from build123d import *

# Parameters (mm, degrees)
EXTRUDE1_DEPTH      = 3.175
SKETCH3_R           = 2.0955
EXTRUDE2_DEPTH      = 4.175
CIRPATTERN1_COUNT   = 10
CIRPATTERN1_ANGLE   = 35
EXTRUDE3_DEPTH      = 1
EXTRUDE3_DEPTH_BACK = 4.175
SKETCH5_W           = 1.778
SKETCH5_H           = 1.961783436
EXTRUDE4_DEPTH      = 4.175


with BuildPart() as part:
    # Sketch1 → Extrude1 (new body)
    with BuildSketch(Plane.XY):
        with BuildLine():
            Line((0, 0), (228.6, 0))
            Line((228.6, 0), (228.6, 90.4875))
            ThreePointArc((228.6, 90.4875), (105.671212021, 67.042793316), (0, 0))
        make_face()
        with BuildLine():
            Line((40.029392194, 9.525), (209.55, 9.525))
            ThreePointArc((209.55, 9.525), (216.285192091, 12.314807909), (219.075, 19.05))
            Line((219.075, 19.05), (219.075, 74.358899247))
            ThreePointArc((219.075, 74.358899247), (218.099794794, 76.648337576), (215.773250164, 77.531368235))
            ThreePointArc((215.773250164, 77.531368235), (122.297861029, 59.693048715), (38.147400573, 15.25709455))
            ThreePointArc((38.147400573, 15.25709455), (37.012821277, 11.709583471), (40.029392194, 9.525))
        make_face(mode=Mode.SUBTRACT)
    extrude(amount=EXTRUDE1_DEPTH)

    # Sketch3 → Extrude2 (cut, through all)
    with BuildSketch(Plane.XY.offset(3.175)):
        with Locations((15.875, 7.775506467)):
            Circle(SKETCH3_R)
    extrude2 = extrude(amount=-EXTRUDE2_DEPTH, mode=Mode.SUBTRACT)

    # CirPattern1: Extrude2 ×10 about axis
    cirpattern1_axis = Axis((228.6, -243.514144737, 0), (0, 0, -1))
    for i in range(1, CIRPATTERN1_COUNT):
        add(extrude2.rotate(cirpattern1_axis, i * CIRPATTERN1_ANGLE / (CIRPATTERN1_COUNT - 1)), mode=Mode.SUBTRACT)

    # Sketch4 → Extrude3 (cut, two sides)
    with BuildSketch(Plane.XY.offset(3.175)) as extrude3_sk:
        with BuildLine():
            Line((726.667212815, 85.4075), (228.6, 85.4075))
            ThreePointArc((228.6, 85.4075), (107.540898152, 62.319375722), (3.476893058, -3.703729831))
            Line((3.476893058, -3.703729831), (-359.654286867, -344.594760291))
            Line((-359.654286867, -344.594760291), (6.971445482, -1270.807136749))
            Line((6.971445482, -1270.807136749), (1093.292945163, -840.804876459))
            Line((1093.292945163, -840.804876459), (726.667212815, 85.4075))
        make_face()
    extrude(amount=EXTRUDE3_DEPTH, mode=Mode.SUBTRACT)
    extrude(extrude3_sk.sketch, amount=-EXTRUDE3_DEPTH_BACK, mode=Mode.SUBTRACT)

    # Sketch5 → Extrude4 (cut, through all)
    with BuildSketch(Plane.XY.offset(3.175)):
        with Locations((224.536, 86.35109773)):
            Rectangle(SKETCH5_W, SKETCH5_H)
    extrude(amount=-EXTRUDE4_DEPTH, mode=Mode.SUBTRACT)


solid = part.part
Can you work these out from the model? Positions are in its coordinate system, mm. Coordinates: 2 decimals unless noted, no trailing zeros. Loops run counter-clockwise (first coordinate to the right, second up) from the corner with the lowest first, then second, coordinate; pieces in that order, holes last. Notation, with made-up numbers: M 49,14 L 79,14 A22 cw 79,22 Z; hole C 61.5,79 d1. An arc over 180 degrees is marked long. Return JSON: item names as keys, results as strings. Group by question number.
Item 1: If I drill on L1, parallel to Y at x = 22, z = 1.8; L2, parallel to Y at x = 114, z = 1.2; L3, parallel to X at y = 55, z = 2.5, over which ranges is the centre line in solid material (lowest first)? Write a range as from..to.
Item 2: I'm going to push flat-ended pins straight in: pin 1 Ø0.5 at (x, z) = (224.5, 2) entering from -Y; pin 2 Ø5.5 at (x, y) = (15.88, 7.78) entering from +Z (3 decimals); pin 3 Ø1 at (y, z) = (46, 2.5) entering from -X. Where does each tip first touch, or does it pass through?
Item 3: Imagine slicing it at A-A (z = 2.65). Please give me the cut outline in (x, y) (1 decimal).
Item 4: Imagine slicing it at B-B (y = 15.5). Please give me the cut outline in (x, z) (3 decimals).
Item 5: Imagine slicing it at C-C (x = 142). Please give me the cut outline in (y, z) (3 decimals), and give its area (3 significant figures).
Verdict:
{
 "1": {"L1": "y = 12.43..18.92", "L2": "y = 64.8..70.21", "L3": "x = 78.78..89.05"},
 "2": {"pin 1": "stops at y = 87.33", "pin 2": "stops at z = 3.175", "pin 3": "stops at x = 61.18"},
 "3": {"outline": "M 0,0 L 7.5,0 A328.9 cw 14.5,6.2 A2.1 cw long 17.7,8.9 A328.9 cw 31.9,20.1 A2.1 cw long 35.3,22.6 A328.9 cw 50.3,32.9 A2.1 cw long 53.8,35.1 A328.9 cw 69.4,44.3 A2.1 cw long 73.1,46.3 A328.9 cw 89.3,54.5 A2.1 cw long 93.1,56.2 A328.9 cw 109.8,63.2 A2.1 cw long 113.7,64.7 A328.9 cw 130.9,70.6 A2.1 cw long 134.9,71.8 A328.9 cw 152.4,76.5 A2.1 cw long 156.5,77.4 A328.9 cw 174.3,80.9 A2.1 cw long 178.4,81.6 A328.9 cw 196.4,83.8 A2.1 cw long 200.6,84.2 A328.9 cw 223.6,85.4 L 223.6,87.3 L 225.4,87.3 L 225.4,85.4 A328.9 cw 228.6,85.4 L 228.6,90.5 A334 ccw Z"},
 "4": {"outline": "M 17.724,0 L 25.866,0 L 25.866,3.175 L 17.724,3.175 Z"},
 "5": {"outline": "M 73.803,0 L 79.065,0 L 79.065,3.175 L 73.803,3.175 Z", "area": "16.7 mm^2"}
}
